Design review of the part built by this model. Coordinates are the model's own, in mm. Face numbers are marked on the shaded views. Coordinates: 2 decimals unless noted, no trailing zeros. Loops run counter-clockwise (first coordinate to the right, second up) from the corner with the lowest first, then second, coordinate; pieces in that order, holes last. Notation, with made-up numbers: M 7.5,72.5 L 43.5,72.5 A29 ccw 43.5,99.5 Z; hole C 82,84 d6. An arc over 180 degrees is marked long. Answer as a JSON object with one key per item and string values. Group by question number.
1. Insertion check: pin 1 (4 mm diameter, centred on x = -15, y = -2, fed in from -Z); pin 2 (3 mm diameter, centred on x = -2.5, y = -5, fed in from +Z); pin 3 (1.5 mm diameter, centred on x = -24, y = -3, fed in from +Z); pin 4 (12 mm diameter, centred on x = -28, z = -17.5, fed in from -Y). Each pin has a flat end and moves straight along its axis. Give the tip position at first contact, or say it passes through.
2. Consider section B-B (z = 0). State the section outline as (x, y) points, then the cut area to 3 significant figures.
3. Consider section C-C (y = -2.75). State the section outline as (x, z) points.
4. Draft analysis for pull direction X (two halves, no side actions). For the marked faces 1 and 2, state which applies: +X half, -X half, draft (parallel to the pull), parting line (faces both ways), or undercut.
5. Consider section A-A (x = 0). State the section outline as (y, z) points.
6. To check wall thickness, follow probe 1 along Z at (x, y) = (0, -3.5); probe 2 along Z at (x, y) = (13.5, -9). State the ranges of each line that lie inside material, in increasing order.
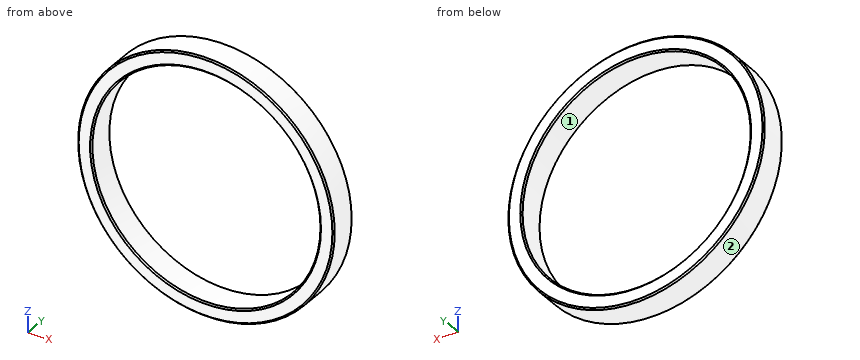
from build123d import *

# Parameters (mm, degrees)
SKETCH_R     = 45
SKETCH_R_2   = 40
PAD_DEPTH    = 10
CHAMFER_SIZE = 0.5


with BuildPart() as part:
    # Sketch → Pad (new body)
    with BuildSketch(Plane.XZ):
        Circle(SKETCH_R)
        Circle(SKETCH_R_2, mode=Mode.SUBTRACT)
    extrude(amount=PAD_DEPTH)

    # Chamfer
    chamfer_edges = [part.edges().sort_by_distance(p)[0] for p in [
        (-45, -10, 0),
        (-40, -10, 0),
        (-45, 0, 0),
        (-40, 0, 0),
    ]]
    chamfer(chamfer_edges, length=CHAMFER_SIZE)


solid = part.part
Findings below:
{
 "1": {"pin 1": "stops at z = -43.08", "pin 2": "stops at z = 44.99", "pin 3": "stops at z = 38.53", "pin 4": "passes through"},
 "2": {"outline": "M -45,-9.5 L -44.5,-10 L -40.5,-10 L -40,-9.5 L -40,-0.5 L -40.5,0 L -44.5,0 L -45,-0.5 Z; M 40,-9.5 L 40.5,-10 L 44.5,-10 L 45,-9.5 L 45,-0.5 L 44.5,0 L 40.5,0 L 40,-0.5 Z", "area": "99.0 mm^2"},
 "3": {"outline": "C 0,0 d90; hole C 0,0 d80"},
 "4": {"face 1": "undercut", "face 2": "parting line"},
 "5": {"outline": "M -10,-44.5 L -9.5,-45 L -0.5,-45 L 0,-44.5 L 0,-40.5 L -0.5,-40 L -9.5,-40 L -10,-40.5 Z; M -10,40.5 L -9.5,40 L -0.5,40 L 0,40.5 L 0,44.5 L -0.5,45 L -9.5,45 L -10,44.5 Z"},
 "6": {"probe 1": "z = -45 to -40, 40 to 45", "probe 2": "z = -42.93 to -37.65, 37.65 to 42.93"}
}
